```python
from build123d import *

# Parameters (mm, degrees)
F0_R     = 5.9
F1_DEPTH = 3.1
F2_R     = 3.09999
F4_DEPTH = 2
F5_R     = 2.5
F6_DEPTH = 8
F7_SIZE  = 0.5


# Not quite as in the source:
# - a fillet or chamfer is up to 0.001 mm smaller than in the source, because OpenCascade refuses the exact size


with BuildPart() as f1:
    # F0 (on Right) → F1 (new body)
    with BuildSketch(Plane.YZ):
        Circle(F0_R)
    extrude(amount=-F1_DEPTH)

    # F2 (radius 3.1 in the source; OpenCascade refuses exactly that, so slightly less here)
    f2_edges = [f1.edges().sort_by_distance(p)[0] for p in [
        (0, -5.9, 0),
    ]]
    fillet(f2_edges, radius=F2_R)

    # F3 (on face) → F4 (cut)
    with BuildSketch(Plane.YZ):
        Polygon((0.5, 2.5), (0, 2.5), (-0.5, 2.5), (-0.5, 0.5), (-2.5, 0.5), (-2.5, 0), (-2.5, -0.5), (-0.5, -0.5), (-0.5, -2.5), (0, -2.5), (0.5, -2.5), (0.5, -0.5), (2.5, -0.5), (2.5, 0), (2.5, 0.5), (0.5, 0.5), align=None)
    extrude(amount=-F4_DEPTH, mode=Mode.SUBTRACT)

    # F5 (on face) → F6 (join)
    with BuildSketch(Plane(origin=(-3.1, 0, 0), x_dir=(0, -1, 0), z_dir=(-1, 0, 0))):
        Circle(F5_R)
    extrude(amount=F6_DEPTH)

    # F7
    f7_edges = [f1.edges().sort_by_distance(p)[0] for p in [
        (-11.1, 2.5, 0),
    ]]
    chamfer(f7_edges, length=F7_SIZE)


solid = f1.part
```
Input: part model. Units: mm. Frame: model coordinates. A direction names the side the tool comes from. Coordinates: 2 decimals unless noted, no trailing zeros. Write each loop counter-clockwise with the first axis right and the second up, starting at its lowest first coordinate (ties: lowest second). Pieces come first, ordered by that corner, then holes. Notation, with made-up numbers: (21, 25.5) -> (78, 25.5) arc R13 ccw to (78, 50.5) -> close; hole circle Ø1 at (8, 63). An arc over 180 degrees is marked (long way). Write each question's results on one line, items separated by ' | '.
Item 1: Set-up query: faces 1 (the flat face through (-1, 1, -0.5)), 2 (the flat face through (-3.1, 0, -3)). Return all of +Z, -Z, +X, -X, +Y, -Y with unobstructed straight access to the full face (end or side cutting, diameter ignored); none if empty.
Conclusion:
face 1: +X | face 2: -X
Item 2: Section query A-A on x = -5.5. Return loops of the section in (y, z).
Conclusion:
outline: circle Ø5 at (0, 0)
Item 3: Pin query (flat end, axial travel): pin 1 Ø1.6 at (x, z) = (-1, -1.5) entering from +Y; pin 2 Ø1 at (x, z) = (-1, -1) entering from -Y; pin 3 Ø5 at (x, z) = (-6, -2) entering from +Y. Return the tip coordinate at first contact, or that it passes through.
Conclusion:
pin 1: stops at y = 5.46 | pin 2: stops at y = -5.37 | pin 3: stops at y = 2.5
Item 4: Material intervals for probe 1 along Y at (x, z) = (-1.75, 0); probe 2 along Y at (x, z) = (-1.5, -2.25); probe 3 along Z at (x, y) = (-1.5, 1.5), sorted ascending.
Conclusion:
probe 1: y = -5.59 to -2.5, 2.5 to 5.59 | probe 2: y = -4.97 to -0.5, 0.5 to 4.97 | probe 3: z = -5.24 to -0.5, 0.5 to 5.24
Item 5: Mould query, pull axis Z, two halves, no side actions, for faces 3 (the flat face through (-11.1, 0, 0)), 4 (the cylindrical face through (-6.8, 0.54, -2.44)), 5 (the flat face through (-1, 0.5, -2)). Classes: +Z half, -Z half, draft (parallel to the pull), parting line (faces both ways), or undercut.
Conclusion:
face 3: draft | face 4: parting line | face 5: undercut
